Model file for the job. Use its own axes, mm. A direction names the side the tool comes from. Give positions to 0.01 mm unless a question says otherwise; leave off trailing zeros. Write each loop counter-clockwise with the first axis right and the second up, starting at its lowest first coordinate (ties: lowest second). Pieces come first, ordered by that corner, then holes. Notation, with made-up numbers: (60.5, 17) - (103.5, 17) arc R12 ccw to (103.5, 40) - close; hole circle Ø7 at (62.25, 31.25). An arc over 180 degrees is marked (long way). One line per item, written item: value. Start each with the question number.
(1) 3-axis set-ups, long thin cutter, end or side, ignore diameter. For faces 1 (the face through (0, 0, 4)), 2 (the face through (2.95, -7.43, 0)): which of +Z, -Z, +X, -X, +Y, -Y reach the whole face in a straight line?
(2) Cut at C-C, the plane z = 2. List the corners of the cut face in (x, y), and give its area (3 significant figures).
(3) Drop flat-ended pins along their axis: P1, Ø2, axis at y = 1, z = -1.5, coming from the +X side; P2, Ø1, axis at y = -2, z = -1, coming from the +X side; P3, Ø4, axis at x = 2.5, z = 3, coming from the -Y side. Give the stop position or say it passes through.
(4) Probe L1, parallel to Z at x = -6.25, y = 5.25; L2, parallel to Y at x = -1.75, z = -1; L3, parallel to Y at x = -3.25, z = 0.5. List the from-to ranges inside material, lowest first.
(5) Cut at A-A, the plane x = 0. List the corners of the cut face in (y, z), and give its area (3 significant figures).
(6) Cut at D-D, the plane z = -1.25. List the corners of the cut face in (x, y).
from build123d import *

# Parameters (mm, degrees)
F0_R     = 10.1
F1_DEPTH = 4
F2_R     = 1.5
F3_R     = 7.8
F4_DEPTH = 4


with BuildPart() as f1:
    # F0 (on Top) → F1 (new body)
    with BuildSketch(Plane.XY):
        Circle(F0_R)
    extrude(amount=F1_DEPTH)

    # F2
    f2_edges = [f1.edges().sort_by_distance(p)[0] for p in [
        (-10.1, 0, 4),
    ]]
    fillet(f2_edges, radius=F2_R)

    # F3 (on face) → F4 (join)
    with BuildSketch(Plane(origin=(0, 0, 0), x_dir=(1, 0, 0), z_dir=(0, 0, -1))):
        Circle(F3_R)
    extrude(amount=F4_DEPTH)


solid = f1.part
Answers follow:
1. face 1: +Z, +X, -X, +Y, -Y
1. face 2: -Z
2. outline: circle Ø20.2 at (0, 0)
2. area: 320 mm²
3. P1: stops at x = 7.8
3. P2: stops at x = 7.65
3. P3: stops at y = -10.08
4. L1: z = 0 to 4
4. L2: y = -7.6 to 7.6
4. L3: y = -9.56 to 9.56
5. outline: (-10.1, 0) - (-7.8, 0) - (-7.8, -4) - (7.8, -4) - (7.8, 0) - (10.1, 0) - (10.1, 2.5) arc R1.5 ccw to (8.6, 4) - (-8.6, 4) arc R1.5 ccw to (-10.1, 2.5) - close
5. area: 142 mm²
6. outline: circle Ø15.6 at (0, 0)
